For this review, take the finished solid that the model builds, in its own axes (mm). Face numbers are marked on the shaded views. A direction names the side the tool comes from. Give positions to 0.01 mm unless a question says otherwise; leave off trailing zeros. Loops run counter-clockwise (first coordinate to the right, second up) from the corner with the lowest first, then second, coordinate; pieces in that order, holes last. Notation, with made-up numbers: (-17, -23) - (-9, -23) arc R30 ccw to (-9, 12) - close; hole circle Ø3 at (15, -13). An arc over 180 degrees is marked (long way). Use CSV: the item, a comma, the result in double quotes. Start each with the question number.
1. Take a section at C-C on y = 9.75. Give the boundary of the cut face in (x, z), plus the area to 3 significant figures.
2. Take a section at B-B on z = -17.5. Give the boundary of the cut face in (x, y).
3. For the marked faces 1 and 2, list the 3-axis set-ups (+Z, -Z, +X, -X, +Y, -Y) from which the entire face can be reached by the end or side of a thin tool; tool diameter is ignored.
4. Wall thickness on line 1 (Z direction, x = 10.5, y = 6.5); line 2 (Y direction, x = 0.25, z = -31.75); line 3 (Y direction, x = 11, z = -31): over which ranges is each line inside the solid? List them lowest first.
5. For pin 1 (6 mm diameter, centred on x = 11.5, y = 4, fed in from +Z); pin 2 (8.5 mm diameter, centred on x = 1.5, z = -24.5, fed in from +Y); pin 3 (1.5 mm diameter, centred on y = 14.5, z = -52, fed in from +X), all flat-tipped, find the tip position at first contact; note any pin that passes through.
6. Take a section at D-D on z = -55.5. Give the boundary of the cut face in (x, y).
7. Take a section at A-A on x = 18.5. Give the boundary of the cut face in (y, z) (3 decimals).
Autodesk Inventor part; units mm, degrees
ref_plane "YZ Plane" through (0, 0, 0) normal (1, 0, 0) x (0, 1, 0)
ref_plane "XZ Plane" through (0, 0, 0) normal (0, 1, 0) x (-1, 0, 0)
ref_plane "XY Plane" through (0, 0, 0) normal (0, 0, 1) x (1, 0, 0)
sketch "Sketch1" plane through (0, 0, 0) normal (0, 0, 1) x (1, 0, 0)
  line L0 (-12.7691, 1.6289) -> (20.2509, 1.6289)
  line L1 (20.2509, 1.6289) -> (20.2509, 7.9789)
  line L2 (20.2509, 7.9789) -> (-6.4191, 7.9789)
  line L3 (-12.7691, 1.6289) -> (-12.7691, 7.9789)
  line L4 (-12.7691, 7.9789) -> (-6.4191, 7.9789)
  point P0 (0, 0)
  dimension "d1" = 6.35
  dimension "d3" = 26.67
extrude "Extrusion1" add sketch "Sketch1" against normal blind 63.5
sketch "Sketch5" plane through (20.2509, 1.6289, 0) normal (1, 0, 0) x (0, 0, -1)
  line L0 (63.5, 0) -> (63.5, 6.35)
  line L1 (0, 0) -> (0, 6.35)
  point P0 (0, -1.6289)
  point P1 (3.556, 3.556)
  point P2 (31.75, 3.556)
  point P3 (59.944, 3.556)
  dimension "d34" = 3.556
  dimension "d35" = 3.556
  dimension "d36" = 31.75
  dimension "d37" = 3.556
hole "Hole3" at (20.2509, 5.1849, -3.556) at (20.2509, 5.1849, -31.75) at (20.2509, 5.1849, -59.944) direction (-1, 0, 0) diameter 3.302 depth 25.4 tip angle 118
sketch "Sketch8" plane through (-12.7691, 7.9789, 0) normal (0, 1, 0) x (1, 0, 0)
  line L0 (33.02, 63.5) -> (0, 63.5)
  line L1 (0, 0) -> (0, 63.5)
  line L2 (33.02, 0) -> (0, 0)
  arc A0 (4.0894, 0) -> (4.0894, 63.5) centre (-222.295, 31.75) ccw
  point P0 (12.7691, 0)
  dimension "d48" = 4.0894
  dimension "d49" = 4.0894
  dimension "d50" = 228.6
extrude "Extrusion3" add sketch "Sketch8" along normal blind 12.7
properties part number "JF-AT-JC0016" material "Aluminum-6061"
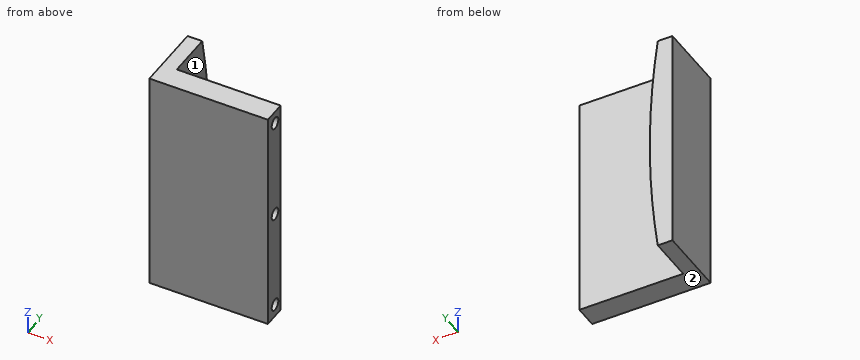
Check result:
1,outline,"(-12.77, -63.5) - (-8.68, -63.5) arc R228.6 ccw to (-8.68, 0) - (-12.77, 0) - close"
1,area,"354 mm²"
2,outline,"(-12.77, 1.63) - (20.25, 1.63) - (20.25, 7.98) - (-6.91, 7.98) - (-6.91, 20.68) - (-12.77, 20.68) - close"
3,face 1,"+X, +Y"
3,face 2,"-Z, +X, -X, +Y, -Y"
4,line 1,"z = -63.5 to -60.94, -58.95 to -32.75, -30.75 to -4.55, -2.56 to 0"
4,line 2,"y = 1.63 to 3.53, 6.84 to 7.98"
4,line 3,"y = 1.63 to 3.71, 6.66 to 7.98"
5,pin 1,"stops at z = 0"
5,pin 2,"stops at y = 7.98"
5,pin 3,"stops at x = -7.3"
6,outline,"(-12.77, 1.63) - (20.25, 1.63) - (20.25, 7.98) - (-7.7, 7.98) - (-7.7, 20.68) - (-12.77, 20.68) - close"
7,outline,"(1.629, -63.5) - (7.979, -63.5) - (7.979, 0) - (1.629, 0) - close; hole circle Ø3.302 at (5.185, -59.944); hole circle Ø3.302 at (5.185, -31.75); hole circle Ø3.302 at (5.185, -3.556)"
